```python
from build123d import *

# Parameters (mm, degrees)
F0_W     = 60
F0_H     = 60
F1_DEPTH = 30
F1_TAPER = 45
F3_W     = 60
F3_H     = 60
F4_DEPTH = 30
F4_TAPER = 45


with BuildPart() as f1:
    # F0 (on Top) → F1 (new body)
    with BuildSketch(Plane.XY):
        Rectangle(F0_W, F0_H)
    extrude(amount=F1_DEPTH, taper=F1_TAPER)

    # F3 (on offset) → F4 (join)
    with BuildSketch(Plane.XY.offset(25)):
        with Locations((0, -6.210045305)):
            Rectangle(F3_W, F3_H)
    extrude(amount=F4_DEPTH, taper=F4_TAPER)


solid = f1.part
```
Read the model definition and answer for the solid it produces. Units are mm, in the model's axes. A direction names the side the tool comes from. Give positions to 0.01 mm unless a question says otherwise; leave off trailing zeros. Order: outer loops, then holes, each group sorted by start corner. A loop starts at its lowest first (then second) coordinate and runs counter-clockwise, first axis right, second up. Notation, with made-up numbers: (73, -14.5) -> (127, -14.5) arc R14 cw to (127, 10.5) -> close; hole circle Ø11 at (3, 60). An arc over 180 degrees is marked (long way). One line per item, written item: value. Start each with the question number.
(1) Straight lines are drawn through the part: L1, parallel to Z at x = 7, y = -24.5; L2, parallel to Z at x = -14, y = -29; L3, parallel to Z at x = 2.5, y = -4.5. For each, find the intervals that lie inside material, in ascending order.
(2) Flat-ended cylindrical pins translate along their axes: P1, Ø2, axis at x = -14.5, z = 37, coming from the -Y side; P2, Ø5, axis at x = -3.5, y = 2, coming from the +Z side; P3, Ø6, axis at x = 16, z = 25, coming from the +Y side. Find the tip coordinate at first contact, or state that the pin passes through.
(3) A tool of negligible diameter and unlimited length cuts with its end or side. For faces 1 (the flat face through (0, -20, 10)), 2 (the flat face through (0.42, -24.75, 36.46)), 3 (the flat face through (20, 0, 10)), from which of +Z, -Z, +X, -X, +Y, -Y can it reach the whole face along a straight path? Write none if from no direction.
(4) For a pull along Z with two mould halves and no side action, classify faces 4 (the flat face through (0, 20, 10)), 5 (the flat face through (0, 0, 0)), 6 (the flat face through (-19, -7, 36)), 7 (the flat face through (-20, 0, 10)) as released by +Z, released by -Z, zero draft, split by the parting line, or undercut.
(5) The part is cut by section B-B (x = 21.5). Determine the outline of the cut face in (y, z), and give its area (4 significant figures).
(6) The part is cut by section C-C (z = 23.5). Determine the outline of the cut face in (x, y).
(7) The part is cut by section A-A (y = -11). Determine the outline of the cut face in (x, z).
(8) The part is cut by section D-D (y = 1). Determine the outline of the cut face in (x, z), and give its area (3 significant figures).
Taken from the geometry:
1. L1: 0 to 5.5, 25 to 36.71
1. L2: 0 to 1, 25 to 32.21
1. L3: 0 to 52.5
2. P1: y = -25.21
2. P2: z = 49.29
2. P3: y = 23.79
3. face 1: +X, -X, -Y
3. face 2: +Z, +X, -X, -Y
3. face 3: +X, +Y, -Y
4. face 4: undercut
4. face 5: released by -Z
4. face 6: released by +Z
4. face 7: undercut
5. outline: (-36.21, 25) -> (23.79, 25) -> (15.29, 33.5) -> (-27.71, 33.5) -> close; (-30, 0) -> (30, 0) -> (21.5, 8.5) -> (-21.5, 8.5) -> close
5. area: 875.5 mm^2
6. outline: (-6.5, -6.5) -> (6.5, -6.5) -> (6.5, 6.5) -> (-6.5, 6.5) -> close
7. outline: (-30, 0) -> (30, 0) -> (11, 19) -> (-11, 19) -> close; (-30, 25) -> (30, 25) -> (4.79, 50.21) -> (-4.79, 50.21) -> close
8. outline: (-30, 0) -> (30, 0) -> (5, 25) -> (30, 25) -> (7.21, 47.79) -> (-7.21, 47.79) -> (-30, 25) -> (-5, 25) -> close
8. area: 1,720 mm^2
